Input: part model. Units: mm. Frame: model coordinates. Face numbers are marked on the shaded views. A direction names the side the tool comes from. Give positions to 0.01 mm unless a question says otherwise; leave off trailing zeros. Write each loop counter-clockwise with the first axis right and the second up, starting at its lowest first coordinate (ties: lowest second). Pieces come first, ordered by that corner, then holes. Notation, with made-up numbers: (53.5, -12) - (107.5, -12) arc R17 ccw to (107.5, 18) - close; hole circle Ø3 at (16.5, 83). An arc over 180 degrees is marked (long way). Answer as CSV lines item,"result".
```python
from build123d import *

# Parameters (mm, degrees)
F0_W     = 76.2
F0_H     = 50.8
F0_R     = 12.7
F1_DEPTH = 12.7
F2_R     = 2.54
F3_T     = 2.54


# Not quite as in the source:
# - a shell that OpenCascade refuses in one call is made with other operations: the cavity is built on its own and cut out


with BuildPart() as f1:
    # F0 (on Top) → F1 (new body)
    with BuildSketch(Plane.XY):
        Rectangle(F0_W, F0_H)
        Circle(F0_R, mode=Mode.SUBTRACT)
    extrude(amount=F1_DEPTH)

    # F2
    f2_edges = [f1.edges().sort_by_distance(p)[0] for p in [
        (-38.1, -25.4, 6.35),
        (38.1, -25.4, 6.35),
        (38.1, 25.4, 6.35),
        (-38.1, 25.4, 6.35),
        (0, 25.4, 12.7),
        (-38.1, 0, 12.7),
        (0, -25.4, 12.7),
        (38.1, 0, 12.7),
        (-12.7, 0, 12.7),
    ]]
    fillet(f2_edges, radius=F2_R)

    # F3: shell of thickness 2.54, made by hand


with BuildPart() as f3_core1:
    # F3_t2: copy of F1
    add(f1.part)

    # the walls: a layer under each face that stays
    f3_faces = [f3_core1.faces().sort_by_distance(p)[0] for p in [
        (38.1, 0, 5.08),
        (0, -25.4, 5.08),
        (0, 25.4, 5.08),
        (-38.1, 0, 5.08),
        (-12.7, 0, 5.08),
        (-23.7066666667, -15.24, 12.7),
    ]]
    thicken(f3_faces, amount=-F3_T, mode=Mode.SUBTRACT)


with BuildPart() as f1_1:
    add(f1.part)

    # what is left inside the walls is the cavity
    f3_cavity = [f3_core1.part.solids().sort_by_distance(p)[0] for p in [
        (-17.78, 7.62, 0.0254),
    ]]
    add(f3_cavity, mode=Mode.SUBTRACT)


solid = f1_1.part
```
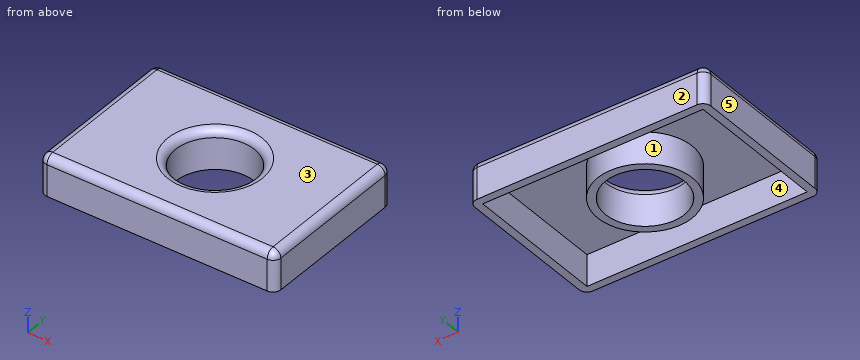
Item 1: Cut plane C-C on y = 0. Return the cut outline in (x, z), plus the area to 3 significant figures.
The answers:
outline,"(-38.1, 0) - (-35.56, 0) - (-35.56, 10.16) - (-15.24, 10.16) - (-15.24, 0) - (-12.7, 0) - (-12.7, 10.16) arc R2.54 ccw to (-15.24, 12.7) - (-35.56, 12.7) arc R2.54 ccw to (-38.1, 10.16) - close; (12.7, 0) - (15.24, 0) - (15.24, 10.16) - (35.56, 10.16) - (35.56, 0) - (38.1, 0) - (38.1, 10.16) arc R2.54 ccw to (35.56, 12.7) - (15.24, 12.7) arc R2.54 ccw to (12.7, 10.16) - close"
area,"227 mm²"
Item 2: Reachability of the marked faces 4 and 5 from +Z, -Z, +X, -X, +Y, -Y: full face, straight path, thin tool, end or side. Return the list, or none.
The answers:
face 4,"-Z"
face 5,"+Z, -Z, -X, +Y, -Y"
Item 3: Contact query for flat-ended pins moving along their axis: pin 1 (1 mm diameter, centred on x = -7, y = -12, fed in from +Z); pin 2 (23 mm diameter, centred on x = 0, y = 0, fed in from -Z). Output: stop coordinate, or through.
The answers:
pin 1,"z = 12.55"
pin 2,"through"
Item 4: Cut plane D-D on x = -31.5. Return the cut outline in (y, z), plus the area to 3 significant figures.
The answers:
outline,"(-25.4, 0) - (-22.86, 0) - (-22.86, 10.16) - (22.86, 10.16) - (22.86, 0) - (25.4, 0) - (25.4, 10.16) arc R2.54 ccw to (22.86, 12.7) - (-22.86, 12.7) arc R2.54 ccw to (-25.4, 10.16) - close"
area,"178 mm²"
Item 5: Cut plane B-B on x = 0. Return the cut outline in (y, z), plus the area to 3 significant figures.
The answers:
outline,"(-25.4, 0) - (-22.86, 0) - (-22.86, 10.16) - (-15.24, 10.16) - (-15.24, 0) - (-12.7, 0) - (-12.7, 10.16) arc R2.54 ccw to (-15.24, 12.7) - (-22.86, 12.7) arc R2.54 ccw to (-25.4, 10.16) - close; (12.7, 0) - (15.24, 0) - (15.24, 10.16) - (22.86, 10.16) - (22.86, 0) - (25.4, 0) - (25.4, 10.16) arc R2.54 ccw to (22.86, 12.7) - (15.24, 12.7) arc R2.54 ccw to (12.7, 10.16) - close"
area,"162 mm²"
Item 6: Cut plane A-A on z = 3.75. Return the cut outline in (x, y), plus the area to 3 significant figures.
The answers:
outline,"(-38.1, -22.86) arc R2.54 ccw to (-35.56, -25.4) - (35.56, -25.4) arc R2.54 ccw to (38.1, -22.86) - (38.1, 22.86) arc R2.54 ccw to (35.56, 25.4) - (-35.56, 25.4) arc R2.54 ccw to (-38.1, 22.86) - close; circle Ø30.48 at (0, 0); hole (-35.56, -22.86) - (35.56, -22.86) - (35.56, 22.86) - (-35.56, 22.86) - close; hole circle Ø25.4 at (0, 0)"
area,"837 mm²"
Item 7: Mould query, pull axis Y, two halves, no side actions, for the marked faces 1, 2 and 3. Classes: +Y half, -Y half, draft (parallel to the pull), parting line (faces both ways), or undercut.
The answers:
face 1,"undercut"
face 2,"+Y half"
face 3,"draft"
Item 8: Ray query, line 1 (Y direction, x = 0, z = 3); line 2 (X direction, y = -16, z = 9.5); line 3 (Y direction, x = -10.5, z = 3). Return the intervals inside material, ascending. Write a range as from..to.
The answers:
line 1,"-25.4..-22.86, -15.24..-12.7, 12.7..15.24, 22.86..25.4"
line 2,"-38.1..-35.56, 35.56..38.1"
line 3,"-25.4..-22.86, -11.05..-7.14, 7.14..11.05, 22.86..25.4"
